Model file for the job. Use its own axes, mm. A direction names the side the tool comes from. Coordinates: 2 decimals unless noted, no trailing zeros. Write each loop counter-clockwise with the first axis right and the second up, starting at its lowest first coordinate (ties: lowest second). Pieces come first, ordered by that corner, then holes.
Q1. Pull direction Z, two halves, no side cores. Call faces 5 (the flat face through (-11, 17, 138)), 6 (the flat face through (-11, 17, 148)), 7 (the flat face through (6, 17, 119)), 8 (the flat face through (-4, 10, 20)): released by +Z, released by -Z, zero draft, split by the parting line, or undercut.
Q2. Band-saw the part on B-B, the plane z = 15. Write the cut outline in (x, y), plus the area to 3 significant figures.
Q3. Pin check, flat tips, straight feed: P1, Ø3, axis at y = 12, z = 48, coming from the +X side; P2, Ø3.5, axis at y = 17.5, z = 123.5, coming from the -X side; P3, Ø6, axis at x = -1.5, z = 112.5, coming from the +Y side. Stop position of each tip, or through.
Q4. Band-saw the part on C-C, the plane y = 17. Write the cut outline in (x, z), plus the area to 3 significant figures.
Q5. Band-saw the part on A-A, the plane y = 0. Write the cut outline in (x, z).
Q6. Which spindle directions (+Z, -Z, +X, -X, +Y, -Y) get a long thin tool onto all of the face, cutting with end or side? Do faces 1 (the flat face through (0, 8.5, 20)), 2 (the flat face through (0, 0, 0)), 3 (the flat face through (3, 15, 178)), 4 (the cylindrical face through (-4.336, -19.524, 118.734)). Say none if no direction does.
Q7. Band-saw the part on D-D, the plane y = -17. Write the cut outline in (x, z).
Q8. Drill centre lines: probe 1 along Y at (x, z) = (0.5, 171); probe 2 along Z at (x, y) = (14, -11.5); probe 3 along Z at (x, y) = (-22, -9). Where is each one in solid material? Low to high.
from build123d import *

# Parameters (mm, degrees)
SKETCH_1_R          = 12.5
EXTRUDE_1_DEPTH     = 40
SKETCH_2_R          = 15
EXTRUDE_2_DEPTH     = 60
SKETCH_3_R          = 20
EXTRUDE_3_DEPTH     = 38
SKETCH_4_R          = 25
EXTRUDE_4_DEPTH     = 10
SKETCH_5_R          = 20
EXTRUDE_5_DEPTH     = 30
SKETCH_6_R          = 15
EXTRUDE_6_DEPTH     = 17
CHAMFER_1_SIZE      = 1
CHAMFER_2_SIZE      = 1
CUT_EXTRUDE_1_DEPTH = 24
CUT_EXTRUDE_2_DEPTH = 14


with BuildPart() as part:
    # 草图1 → 凸台-拉伸1 (new body)
    with BuildSketch(Plane.XY):
        Circle(SKETCH_1_R)
    extrude(amount=EXTRUDE_1_DEPTH)

    # 草图2 → 凸台-拉伸2 (add)
    with BuildSketch(Plane.XY.offset(40)):
        Circle(SKETCH_2_R)
    extrude(amount=EXTRUDE_2_DEPTH)

    # 草图3 → 凸台-拉伸3 (add)
    with BuildSketch(Plane.XY.offset(100)):
        Circle(SKETCH_3_R)
    extrude(amount=EXTRUDE_3_DEPTH)

    # 草图4 → 凸台-拉伸4 (add)
    with BuildSketch(Plane.XY.offset(138)):
        Circle(SKETCH_4_R)
    extrude(amount=EXTRUDE_4_DEPTH)

    # 草图5 → 凸台-拉伸5 (add)
    with BuildSketch(Plane.XY.offset(148)):
        Circle(SKETCH_5_R)
    extrude(amount=EXTRUDE_5_DEPTH)

    # 草图6 → 凸台-拉伸6 (add)
    with BuildSketch(Plane.XY.offset(178)):
        Circle(SKETCH_6_R)
    extrude(amount=EXTRUDE_6_DEPTH)

    # 倒角1
    chamfer_1_edges = [part.edges().sort_by_distance(p)[0] for p in [
        (-15, 0, 195),
    ]]
    chamfer(chamfer_1_edges, length=CHAMFER_1_SIZE)

    # 倒角2
    chamfer_2_edges = [part.edges().sort_by_distance(p)[0] for p in [
        (-12.5, 0, 0),
    ]]
    chamfer(chamfer_2_edges, length=CHAMFER_2_SIZE)

    # 草图7 → 切除-拉伸1 (cut)
    with BuildSketch(Plane(origin=(0, 15, 0), x_dir=(1, 0, 0), z_dir=(0, 1, 0))):
        with BuildLine():
            Line((-6, -131), (-6, -107))
            ThreePointArc((-6, -107), (0, -101), (6, -107))
            Line((6, -107), (6, -131))
            ThreePointArc((6, -131), (0, -137), (-6, -131))
        make_face()
    extrude(amount=CUT_EXTRUDE_1_DEPTH, mode=Mode.SUBTRACT)

    # 草图8 → 切除-拉伸2 (cut)
    with BuildSketch(Plane(origin=(0, 8.5, 0), x_dir=(1, 0, 0), z_dir=(0, 1, 0))):
        with BuildLine():
            Line((-4, -6), (-4, -34))
            ThreePointArc((-4, -34), (0, -38), (4, -34))
            Line((4, -34), (4, -6))
            ThreePointArc((4, -6), (0, -2), (-4, -6))
        make_face()
    extrude(amount=CUT_EXTRUDE_2_DEPTH, mode=Mode.SUBTRACT)


solid = part.part
Answer sheet:
1. face 5: released by -Z
1. face 6: released by +Z
1. face 7: undercut
1. face 8: undercut
2. outline: (-4, 8.5) - (-4, 11.84) arc R12.5 ccw (long way) to (4, 11.84) - (4, 8.5) - close
2. area: 461 mm2
3. P1: stops at x = 10.71
3. P2: stops at x = -12.33
3. P3: stops at y = 15
4. outline: (-18.33, 138) - (-10.54, 138) - (-10.54, 100) - (10.54, 100) - (10.54, 138) - (18.33, 138) - (18.33, 148) - (10.54, 148) - (10.54, 178) - (-10.54, 178) - (-10.54, 148) - (-18.33, 148) - close; hole (-6, 107) arc R6 ccw to (6, 107) - (6, 131) arc R6 ccw to (-6, 131) - close
4. area: 1,400 mm2
5. outline: (-25, 138) - (-20, 138) - (-20, 100) - (-15, 100) - (-15, 40) - (-12.5, 40) - (-12.5, 1) - (-11.5, 0) - (11.5, 0) - (12.5, 1) - (12.5, 40) - (15, 40) - (15, 100) - (20, 100) - (20, 138) - (25, 138) - (25, 148) - (20, 148) - (20, 178) - (15, 178) - (15, 194) - (14, 195) - (-14, 195) - (-15, 194) - (-15, 178) - (-20, 178) - (-20, 148) - (-25, 148) - close
6. face 1: +Y
6. face 2: -Z, +X, -X, +Y, -Y
6. face 3: +Z
6. face 4: -Z
7. outline: (-18.33, 138) - (-10.54, 138) - (-10.54, 100) - (10.54, 100) - (10.54, 138) - (18.33, 138) - (18.33, 148) - (10.54, 148) - (10.54, 178) - (-10.54, 178) - (-10.54, 148) - (-18.33, 148) - close
8. probe 1: y = -19.99 to 19.99
8. probe 2: z = 100 to 178
8. probe 3: z = 138 to 148
